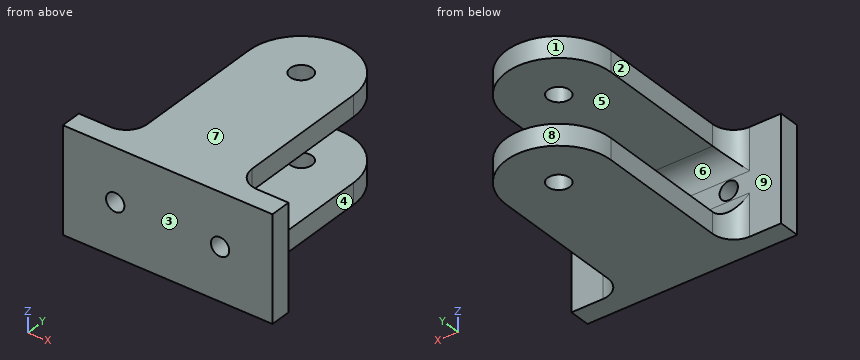
```python
from build123d import *

# Parameters (mm, degrees)
SKETCH1_W            = 76.2
SKETCH1_H            = 38.1
SKETCH1_R            = 3.3274
BOSS_EXTRUDE1_DEPTH  = 7.62
SKETCH2_R            = 4
BOSS_EXTRUDE2_DEPTH  = 7.62
FILLET1_R            = 7.62
FILLET1_OF_MIRROR2_R = 7.62


with BuildPart() as part:
    # Sketch1 → Boss-Extrude1 (new body)
    with BuildSketch(Plane(origin=(0, 0, 0), x_dir=(1, 0, 0), z_dir=(0, 1, 0))):
        with Locations((38.1, 19.05)):
            Rectangle(SKETCH1_W, SKETCH1_H)
        with Locations(Location((19.05, 19.05, 0), (0, 0, 270))):
            Circle(SKETCH1_R, mode=Mode.SUBTRACT)
        with Locations(Location((57.15, 19.05, 0), (0, 0, 90))):
            Circle(SKETCH1_R, mode=Mode.SUBTRACT)
    extrude(amount=BOSS_EXTRUDE1_DEPTH)

    # Sketch2 → Boss-Extrude2 (add)
    with BuildSketch(Plane.XY):
        with BuildLine():
            Line((19.05, 0), (19.05, 63.5))
            ThreePointArc((19.05, 63.5), (38.1, 82.55), (57.15, 63.5))
            Line((57.15, 63.5), (57.15, 0))
            Line((57.15, 0), (19.05, 0))
        make_face()
        with Locations((38.1, 63.5)):
            Circle(SKETCH2_R, mode=Mode.SUBTRACT)
    boss_extrude2 = extrude(amount=-BOSS_EXTRUDE2_DEPTH)

    # Fillet1
    fillet1_edges = [part.edges().sort_by_distance(p)[0] for p in [
        (19.05, 7.62, -3.81),
        (57.15, 7.62, -3.81),
        (38.1, 7.62, -7.62),
    ]]
    fillet(fillet1_edges, radius=FILLET1_R)

    # Mirror2: Boss-Extrude2 across plane
    add(boss_extrude2.mirror(Plane.XY.offset(-19.05)))

    # Fillet1 of Mirror2
    fillet1_of_mirror2_edges = [part.edges().sort_by_distance(p)[0] for p in [
        (19.05, 7.62, -34.29),
        (57.15, 7.62, -34.29),
        (38.1, 7.62, -30.48),
    ]]
    fillet(fillet1_of_mirror2_edges, radius=FILLET1_OF_MIRROR2_R)


solid = part.part
```
Geometry check sheet. Reference: the model listing, model coordinates, mm. Face numbers are marked on the shaded views. A direction names the side the tool comes from. Give positions to 0.01 mm unless a question says otherwise; leave off trailing zeros. Write each loop counter-clockwise with the first axis right and the second up, starting at its lowest first coordinate (ties: lowest second). Pieces come first, ordered by that corner, then holes. Notation, with made-up numbers: (18.5, -16.75) - (63.5, -16.75) arc R17 cw to (63.5, 0.25) - close; hole circle Ø5 at (36.5, 20.25). An arc over 180 degrees is marked (long way). Use a Markdown table: item, result.
Q1. Go/stop test with flat-tipped pins: P1, Ø8.5, axis at y = 38.5, z = -34, coming from the +X side; P2, Ø8.5, axis at y = 36, z = -4.5, coming from the -X side; P3, Ø10, axis at y = 25.5, z = -15, coming from the +X side; P4, Ø11.5, axis at x = 36.5, z = -10.5, coming from the +Y side. Record where each tip stops, or that it passes through.
Computed:
| item | result |
|---|---|
| P1 | stops at x = 57.15 |
| P2 | stops at x = 19.05 |
| P3 | passes through |
| P4 | stops at y = 82.55 |
Q2. Section check C-C, the plane z = -19.05. Enter the section's corners in (x, y), then the cut area to 3 significant figures.
Computed:
| item | result |
|---|---|
| outline | (0, 0) - (15.72, 0) - (15.72, 7.62) - (0, 7.62) - close; (22.38, 0) - (53.82, 0) - (53.82, 7.62) - (22.38, 7.62) - close; (60.48, 0) - (76.2, 0) - (76.2, 7.62) - (60.48, 7.62) - close |
| area | 479 mm² |
Q3. Section check A-A, the plane z = -4.5. Enter the section's corners in (x, y), then the cut area to 3 significant figures.
Computed:
| item | result |
|---|---|
| outline | (0, 0) - (76.2, 0) - (76.2, 7.62) - (64.77, 7.62) arc R7.62 cw to (57.15, 15.24) - (57.15, 63.5) arc R19.05 ccw to (19.05, 63.5) - (19.05, 15.24) arc R7.62 cw to (11.43, 7.62) - (0, 7.62) - close; hole circle Ø8 at (38.1, 63.5) |
| area | 3,250 mm² |
Q4. Thickness scan on L1, parallel to X at y = 3.25, z = -19.05; L2, parallel to Y at x = 38.1, z = -33.5; L3, parallel to Z at x = 52.5, y = 55.5. Record the ranges inside material, lowest first. Write a range as [from, to].
Computed:
| item | result |
|---|---|
| L1 | x = [0, 15.72], [22.38, 53.82], [60.48, 76.2] |
| L2 | y = [0, 59.5], [67.5, 82.55] |
| L3 | z = [-38.1, -30.48], [-7.62, 0] |
Q5. Section check D-D, the plane x = 72.5. Enter the section's corners in (y, z), then the cut area to 3 significant figures.
Computed:
| item | result |
|---|---|
| outline | (0, -38.1) - (7.62, -38.1) - (7.62, 0) - (0, 0) - close |
| area | 290 mm² |
Q6. Section check B-B, the plane y = 71.5. Enter the section's corners in (x, z), then the cut area to 3 significant figures.
Computed:
| item | result |
|---|---|
| outline | (20.81, -38.1) - (55.39, -38.1) - (55.39, -30.48) - (20.81, -30.48) - close; (20.81, -7.62) - (55.39, -7.62) - (55.39, 0) - (20.81, 0) - close |
| area | 527 mm² |
Q7. Set-up check for the marked faces 1, 2, 3, 4 and 5: record each of +Z, -Z, +X, -X, +Y, -Y from which the full face is reachable in a straight line by a thin tool's end or side.
Computed:
| item | result |
|---|---|
| face 1 | +Z, -Z, +Y |
| face 2 | +Z, -Z, -X, +Y |
| face 3 | +Z, -Z, +X, -X, -Y |
| face 4 | +Z, -Z, +X, +Y |
| face 5 | +X, -X, +Y |
Q8. Draft check along Z on the marked faces 6, 7, 8 and 9. Enter one of: pulls with the +Z half, pulls with the -Z half, needs draft (parallel to the pull), parting line crosses it, or undercut.
Computed:
| item | result |
|---|---|
| face 6 | undercut |
| face 7 | pulls with the +Z half |
| face 8 | needs draft |
| face 9 | undercut |
